Model file for the job. Use its own axes, mm. A direction names the side the tool comes from. Give positions to 0.01 mm unless a question says otherwise; leave off trailing zeros. Order: outer loops, then holes, each group sorted by start corner. A loop starts at its lowest first (then second) coordinate and runs counter-clockwise, first axis right, second up. Notation, with made-up numbers: (-14, -12) - (-7, -12) arc R16 cw to (-7, -7) - close; hole circle Ø11 at (41, 37.5). An arc over 180 degrees is marked (long way). Use CSV: the item, a comma, the result in double quotes. Start each with the question number.
(1) Probe L1, parallel to X at y = 6, z = 15; L2, parallel to Z at x = 30, y = 7.4; L3, parallel to Y at x = 28, z = 17.5. List the from-to ranges inside material, lowest first.
(2) Band-saw the part on D-D, the plane z = 14. Give the cut face in (x, y), then the cut area to 3 significant figures.
(3) Drop flat-ended pins along their axis: pin 1 Ø6 at (x, z) = (33.5, 13) entering from +Y; pin 2 Ø5 at (x, y) = (36, 23) entering from +Z; pin 3 Ø10 at (y, z) = (18, 12) entering from -X; pin 4 Ø7.5 at (y, z) = (5.5, -8) entering from +X. Give the stop position or say it passes through.
(4) Band-saw the part on A-A, the plane z = -0.5. Give the cut face in (x, y), then the cut area to 3 significant figures.
(5) Tool access for faces 5 (the flat face through (34, 6, -6)), 6 (the flat face through (31, 35, -6)), 7 (the flat face through (32.1, 10, 12.6)), 8 (the flat face through (20, 30, 10)), 9 (the flat face through (40, 29, 10)): list every direction of +Z, -Z, +X, -X, +Y, -Y with a clear straight run to the whole face (end or side of a thin tool).
(6) Band-saw the part on C-C, the plane y = 33.5. Give the cut face in (x, z), then the cut area to 3 significant figures.
(7) Band-saw the part on B-B, the plane x = 29. Give the cut face in (y, z).
(8) Pull direction Y, two halves, no side cores. Call faces 1 (the cylindrical face through (23.01, 29.46, 22.15)), 2 (the flat face through (30, 20, 5)), 3 (the flat face through (32.1, 27, 12.6)), 4 (the flat face through (30.2, 37, 0.2)): +Y half, -Y half, draft (parallel to the pull), parting line (faces both ways), or undercut.
Autodesk Inventor part; units mm, degrees
ref_plane "YZ Plane" through (0, 0, 0) normal (1, 0, 0) x (0, 1, 0)
ref_plane "XZ Plane" through (0, 0, 0) normal (0, 1, 0) x (-1, 0, 0)
ref_plane "XY Plane" through (0, 0, 0) normal (0, 0, 1) x (1, 0, 0)
sketch "Sketch1" plane through (0, 0, 0) normal (0, 0, 1) x (1, 0, 0)
  line L0 (0, 0) -> (60, 0)
  line L1 (60, 0) -> (60, 37)
  line L2 (60, 37) -> (0, 37)
  line L3 (0, 37) -> (0, 0)
  dimension "d0" = 60
  dimension "d1" = 37
extrude "Extrusion1" add sketch "Sketch1" along normal blind 5
sketch "Sketch2" plane through (0, 0, 5) normal (0, 0, 1) x (1, 0, 0)
  line L0 (20, 27) -> (40, 27)
  line L1 (40, 27) -> (40, 32)
  line L2 (40, 32) -> (20, 32)
  line L3 (20, 32) -> (20, 27)
  line L4 (20, 10) -> (40, 10)
  line L5 (40, 10) -> (40, 5)
  line L6 (40, 5) -> (20, 5)
  line L7 (20, 5) -> (20, 10)
  point P0 (0, 0)
  dimension "d6" = 20
  dimension "d7" = 5
  dimension "d8" = 20
  dimension "d9" = 5
extrude "Extrusion2" add sketch "Sketch2" along normal blind 20
sketch "Sketch3" plane through (20, 32, 5) normal (0, 1, 0) x (1, 0, 0)
  circle A0 centre (10, -10) radius 2.7
  point P0 (-20, 5)
  dimension "d12" = 5.4
extrude "Extrusion3" cut sketch "Sketch3" against normal blind 20
sketch "Sketch4" plane through (20, 10, 5) normal (0, 1, 0) x (1, 0, 0)
  circle A0 centre (10, -10) radius 2.7
  point P0 (-20, 5)
  dimension "d15" = 5.4
extrude "Extrusion4" cut sketch "Sketch4" against normal blind 20
fillet "Fillet1" radius 10 1 edges at (40, 29.5, 25)
fillet "Fillet2" radius 10 1 edges at (20, 29.5, 25)
fillet "Fillet3" radius 10 1 edges at (40, 7.5, 25)
fillet "Fillet4" radius 10 1 edges at (20, 7.5, 25)
sketch "Sketch5" plane through (0, 0, 5) normal (0, 0, 1) x (1, 0, 0)
  circle A0 centre (10, 10) radius 2.5
  circle A1 centre (50, 10) radius 2.5
  circle A2 centre (10, 27) radius 2.5
  circle A3 centre (50, 27) radius 2.5
  point P0 (0, 0)
  dimension "d22" = 5
  dimension "d23" = 5
  dimension "d24" = 5
  dimension "d25" = 5
extrude "Extrusion5" cut sketch "Sketch5" against normal blind 20
fillet "Fillet5" radius 10 1 edges at (0, 37, 2.5)
fillet "Fillet6" radius 10 1 edges at (60, 37, 2.5)
fillet "Fillet7" radius 10 1 edges at (60, 0, 2.5)
fillet "Fillet8" radius 10 1 edges at (0, 0, 2.5)
sketch "Sketch6" plane through (0, 0, 0) normal (0, 0, -1) x (-1, 0, 0)
  point P0 (0, 0)
sketch "Sketch7" plane through (0, 0, 5) normal (0, 0, 1) x (1, 0, 0)
  line L0 (10, 0) -> (50, 0)
  line L1 (50, 37) -> (10, 37)
  line L2 (18, 0) -> (42, 0)
  line L3 (42, 0) -> (42, 37)
  line L4 (42, 37) -> (18, 37)
  line L5 (18, 37) -> (18, 0)
  line L6 (18, 0) -> (0, 0)
  line L7 (0, 0) -> (0, 37)
  line L8 (0, 37) -> (18, 37)
  line L9 (18, 37) -> (18, 0)
  line L10 (42, 0) -> (60, 0)
  line L11 (60, 0) -> (60, 37)
  line L12 (60, 37) -> (42, 37)
  line L13 (42, 37) -> (42, 0)
  dimension "d32" = 24
extrude "Extrusion6" cut sketch "Sketch7" against normal blind 10 contours L6 L7 L8 L1 L5 L0 | L3 L1 L12 L11 L10 L0
sketch "Sketch8" plane through (0, 0, 0) normal (0, 0, -1) x (-1, 0, 0)
  point P0 (0, 0)
sketch "Sketch9" plane through (0, 0, 0) normal (0, 0, -1) x (-1, 0, 0)
  line L0 (-18, 0) -> (-42, 0)
  line L1 (-34, 0) -> (-31, 0)
  line L2 (-31, 0) -> (-31, 9)
  line L3 (-31, 9) -> (-34, 9)
  line L4 (-34, 9) -> (-34, 0)
  line L5 (-18, 0) -> (-18, 37)
  point P0 (0, 0)
  point P1 (-23, 0)
  point P2 (-37, 0)
  point P3 (-18, 5)
  point P4 (-18, 32)
  dimension "d36" = 3
  dimension "d37" = 9
  dimension "d38" = 16
sketch "Sketch10" plane through (0, 0, 0) normal (0, 0, -1) x (-1, 0, 0)
  line L0 (-42, 37) -> (-18, 37)
  line L1 (-34, 37) -> (-31, 37)
  line L2 (-31, 37) -> (-31, 32)
  line L3 (-31, 32) -> (-34, 32)
  line L4 (-34, 32) -> (-34, 37)
  line L5 (-18, 0) -> (-18, 37)
  point P0 (0, 0)
  dimension "d39" = 3
  dimension "d40" = 5
  dimension "d41" = 16
sketch "Sketch11" plane through (0, 0, 0) normal (0, 0, -1) x (-1, 0, 0)
  point P0 (0, 0)
sketch "Sketch12" plane through (0, 0, 5) normal (0, 0, 1) x (1, 0, 0)
  point P0 (0, 0)
sketch "Sketch13" plane through (0, 0, 5) normal (0, 0, 1) x (1, 0, 0)
  point P0 (0, 0)
sketch "Sketch14" plane through (0, 0, 5) normal (0, 0, 1) x (1, 0, 0)
  line L0 (42, 0) -> (42, 37)
  line L1 (18, 0) -> (18, 37)
  line L2 (42, 0) -> (18, 0)
  line L3 (18, 0) -> (18, 2)
  line L4 (18, 2) -> (42, 2)
  line L5 (42, 2) -> (42, 0)
  point P0 (0, 0)
  dimension "d42" = 2
extrude "Extrusion7" add sketch "Sketch10" along normal blind 12
extrude "Extrusion8" add sketch "Sketch9" along normal blind 12
extrude "Extrusion9" cut sketch "Sketch14" against normal blind 22
properties part number "sail_hold_1"
Answer block:
1,L1,"x = 20 to 27.3, 32.7 to 40"
1,L2,"z = 0 to 12.3, 17.7 to 25"
1,L3,"y = 5 to 10, 27 to 32"
2,outline,"(20, 5) - (27.49, 5) - (27.49, 10) - (20, 10) - close; (20, 27) - (27.49, 27) - (27.49, 32) - (20, 32) - close; (32.51, 5) - (40, 5) - (40, 10) - (32.51, 10) - close; (32.51, 27) - (40, 27) - (40, 32) - (32.51, 32) - close"
2,area,"150 mm2"
3,pin 1,"stops at y = 32"
3,pin 2,"stops at z = 5"
3,pin 3,"passes through"
3,pin 4,"stops at x = 34"
4,outline,"(31, 2) - (34, 2) - (34, 9) - (31, 9) - close; (31, 32) - (34, 32) - (34, 37) - (31, 37) - close"
4,area,"36.0 mm2"
5,face 5,"-Z, +X, +Y, -Y"
5,face 6,"-Z, -X, +Y, -Y"
5,face 7,"+Z, +X, -X"
5,face 8,"+Z, -X, +Y, -Y"
5,face 9,"+Z, +X, +Y, -Y"
6,outline,"(18, 0) - (31, 0) - (31, -12) - (34, -12) - (34, 0) - (42, 0) - (42, 5) - (18, 5) - close"
6,area,"156 mm2"
7,outline,"(2, 0) - (37, 0) - (37, 5) - (32, 5) - (32, 12.49) - (27, 12.49) - (27, 5) - (10, 5) - (10, 12.49) - (5, 12.49) - (5, 5) - (2, 5) - close; (5, 17.51) - (10, 17.51) - (10, 24.95) - (5, 24.95) - close; (27, 17.51) - (32, 17.51) - (32, 24.95) - (27, 24.95) - close"
8,face 1,"draft"
8,face 2,"undercut"
8,face 3,"undercut"
8,face 4,"+Y half"
